Check sheet for the modelled part. Datum: model origin and axes. Units: mm. A direction names the side the tool comes from. Round coordinates to 2 decimals unless told otherwise and drop trailing zeros. Write each loop counter-clockwise with the first axis right and the second up, starting at its lowest first coordinate (ties: lowest second). Pieces come first, ordered by that corner, then holes. Notation, with made-up numbers: (63, 78.5) -> (84, 78.5) arc R22 cw to (84, 84.5) -> close; hole circle Ø4 at (22, 1). An arc over 180 degrees is marked (long way). Write item = value, one per line.
Autodesk Inventor part; units mm, degrees
ref_plane "Work Plane1" through (0, 0, -15) normal (0, 0, 1) x (1, 0, 0)
ref_plane "YZ Plane" through (0, 0, 0) normal (1, 0, 0) x (0, 1, 0)
ref_plane "XZ Plane" through (0, 0, 0) normal (0, 1, 0) x (-1, 0, 0)
sketch "Sketch1" plane through (0, 0, 0) normal (0, 0, 1) x (1, 0, 0)
  line L0 (0, 0) -> (25, 0)
  line L1 (25, 0) -> (25, 40)
  line L2 (25, 40) -> (0, 40)
  line L3 (0, 40) -> (0, 0)
  dimension "d1" = 25
  dimension "d2" = 40
  dimension "d3" = 25
extrude "Extrusion1" add sketch "Sketch1" against normal blind 30
sketch "Sketch2" plane through (25, 0, 0) normal (1, 0, 0) x (0, 0, -1)
  line L0 (0, 0) -> (30, 0)
  circle A0 centre (15, 6.56) radius 2.46
extrude "Extrusion2" cut sketch "Sketch2" against normal blind 30
sketch "Sketch3" plane through (0, 0, 0) normal (-1, 0, 0) x (0, 0, 1)
  line L0 (0, 0) -> (-30, 0)
  line L1 (-25.05, 0) -> (-4.95, 0)
  line L2 (-4.95, 0) -> (-4.95, 33.12)
  line L3 (-4.95, 33.12) -> (-25.05, 33.12)
  line L4 (-25.05, 33.12) -> (-25.05, 0)
  dimension "d11" = 20.1
extrude "Extrusion3" cut sketch "Sketch3" against normal blind 20
sketch "Sketch4" plane through (0, 0, 0) normal (0, -1, 0) x (1, 0, 0)
  line L0 (20, -4.95) -> (20, -25.05)
  line L1 (20, -15) -> (25, -15)
  line L2 (25, 0) -> (25, -30)
  line L3 (20, -8.025) -> (25, -8.025)
  line L4 (25, -8.025) -> (25, -21.975)
  line L5 (25, -21.975) -> (20, -21.975)
  line L6 (20, -21.975) -> (20, -8.025)
  line L7 (20, -8.025) -> (25, -21.975) construction
  line L8 (25, -8.025) -> (20, -21.975) construction
  line L9 (25, -12.54) -> (25, -17.46)
  point P0 (0, 0)
  point P1 (22.5, -15)
  dimension "d14" = 13.95
extrude "Extrusion4" add sketch "Sketch4" along normal blind 15
sketch "Sketch5" plane through (20, 0, 0) normal (-1, 0, 0) x (0, 0, 1)
  circle A0 centre (-15, 6.56) radius 2.46
  circle A1 centre (-15, 6.56) radius 4.7025
  circle A2 centre (-15, 6.56) radius 2.46
  circle A3 centre (-15, 6.56) radius 2.46
  point P0 (0, 0)
  dimension "d17" = 9.405
extrude "Extrusion5" cut sketch "Sketch5" against normal blind 2.1
sketch "Sketch6" plane through (25, 0, 0) normal (1, 0, 0) x (0, 0, -1)
  circle A0 centre (15, 6.56) radius 4.7025
  line L0 (15, 6.56) -> (15, 23.56)
  circle A1 centre (15, 23.56) radius 2.46
  point P0 (0, 0)
  dimension "d20" = 17
  dimension "d21" = 4.92
extrude "Extrusion6" cut sketch "Sketch6" against normal blind 10 contours A1
sketch "Sketch7" plane through (20, 0, 0) normal (-1, 0, 0) x (0, 0, 1)
  circle A0 centre (-15, 23.56) radius 2.46
  circle A1 centre (-15, 23.56) radius 4.7025
  point P0 (0, 0)
  dimension "d24" = 9.405
extrude "Extrusion7" cut sketch "Sketch7" against normal blind 2.1
sketch "Sketch9" plane through (25, 0, 0) normal (1, 0, 0) x (0, 0, -1)
  circle A0 centre (15, 6.56) radius 2.46
  circle A1 centre (15, 6.56) radius 2.46
  circle A2 centre (15, 23.56) radius 2.46
  circle A3 centre (15, 23.56) radius 2.46
  line L0 (30, 40) -> (30, 0)
  line L1 (30, 0) -> (30, 40)
  line L2 (30, 40) -> (0, 40)
  line L3 (0, 40) -> (0, 0)
  line L4 (0, 0) -> (8.025, 0)
  line L5 (21.975, 0) -> (21.975, -15)
  line L6 (21.975, -15) -> (8.025, -15)
  line L7 (8.025, -15) -> (8.025, 0)
  line L8 (0, 0) -> (8.025, 0)
  line L9 (21.975, 0) -> (30, 0)
extrude "Extrusion8" add sketch "Sketch9" along normal blind 5
sketch "Sketch10" plane through (0, 40, 0) normal (0, 1, 0) x (1, 0, 0)
  line L0 (0, 30) -> (30, 30)
  line L1 (30, 0) -> (0, 0)
  line L2 (0, 30) -> (30, 30)
  line L3 (30, 30) -> (30, 0)
  line L4 (30, 0) -> (0, 0)
  line L5 (0, 0) -> (0, 30)
extrude "Extrusion9" add sketch "Sketch10" along normal blind 30
sketch "Sketch12" plane through (30, 0, 0) normal (1, 0, 0) x (0, 0, -1)
  circle A0 centre (15, 6.56) radius 2.46
  line L0 (15, 6.56) -> (15, 15.06)
  circle A1 centre (15, 15.06) radius 2.525
  point P0 (0, 0)
  dimension "d31" = 8.5
  dimension "d33" = 5.05
extrude "Extrusion10" cut sketch "Sketch12" against normal blind 30 contours A1
sketch "Sketch15" plane through (0, 0, -25.05) normal (-1, 0, 0) x (0, 0, 1)
  line L0 (0, 33.12) -> (20.1, 33.12)
  line L1 (20.1, 33.12) -> (20.1, 0)
  line L2 (0, 33.12) -> (20.1, 33.12)
  line L3 (20.1, 33.12) -> (20.1, 31.1)
  line L4 (20.1, 31.1) -> (0, 31.1)
  line L5 (0, 31.1) -> (0, 33.12)
  point P0 (25.05, 0)
  dimension "d57" = 2.02
extrude "Extrusion13" add sketch "Sketch15" against normal blind 20
sketch "Sketch17" plane through (0, 0, 0) normal (0, 0, 1) x (1, 0, 0)
  line L0 (0, 70) -> (30, 70)
  line L1 (30, 70) -> (50.0622, 90.0622)
  line L2 (30, 70) -> (80, 70) construction
  line L3 (11.9522, 97.2454) -> (0, 85.2932)
  line L4 (0, 70) -> (0, 85.2932)
  line L5 (0, 70) -> (0, 0)
  line L6 (0, 70) -> (30, 70)
  line L7 (10.923, 112.2849) -> (0, 120.567)
  line L8 (50.0622, 105.3553) -> (50.0622, 120.567)
  line L9 (50.0622, 105.3553) -> (50.0622, 90.0622)
  arc A0 (11.9522, 97.2454) -> (10.923, 112.2849) centre (4.8811, 104.3165) ccw
  line L10 (4, 138.567) -> (0, 140.567)
  line L11 (4, 122.567) -> (0, 120.567)
  line L12 (4, 122.567) -> (8, 130.567)
  line L13 (4, 138.567) -> (8, 130.567)
  line L14 (0, 140.567) -> (30, 140.567)
  line L15 (30, 140.567) -> (50.0622, 120.567)
  dimension "d61" = 45
  dimension "d62" = 32.0271
  dimension "d72" = 10
extrude "Extrusion14" add sketch "Sketch17" against normal blind 30
sketch "Sketch21" plane through (0, 0, 0) normal (0, 0, 1) x (1, 0, 0)
  line L0 (50.0622, 90.0622) -> (30, 70)
  line L1 (30, 70) -> (50.0622, 90.0622)
  line L2 (50.0622, 90.0622) -> (50.0622, 120.567)
  line L3 (50.0622, 90.0622) -> (50.0622, 120.567)
  line L4 (0, 140.567) -> (30, 140.567)
  line L5 (50.0622, 120.567) -> (30, 140.567)
  line L6 (30, 140.567) -> (0, 140.567)
  line L7 (4, 138.567) -> (0, 140.567)
  line L8 (0, 140.567) -> (4, 138.567)
  line L9 (8, 130.567) -> (4, 138.567)
  line L10 (4, 138.567) -> (8, 130.567)
  line L11 (4, 122.567) -> (8, 130.567)
  line L12 (8, 130.567) -> (4, 122.567)
  line L13 (0, 120.567) -> (4, 122.567)
  line L14 (4, 122.567) -> (0, 120.567)
  line L15 (10.923, 112.2849) -> (0, 120.567)
  line L16 (0, 120.567) -> (10.923, 112.2849)
  line L17 (0, 85.2932) -> (11.9522, 97.2454)
  line L18 (11.9522, 97.2454) -> (0, 85.2932)
  line L19 (0, 85.2932) -> (0, 55.2932)
  line L20 (0, 55.2932) -> (30, 55.2932)
  line L21 (30, 55.2932) -> (30, 70)
  arc A0 (11.9522, 97.2454) -> (10.923, 112.2849) centre (4.8811, 104.3165) ccw
  dimension "d79" = 30
  dimension "d81" = 30
extrude "Extrusion15" add sketch "Sketch21" along normal blind 30
ref_plane "Work Plane1" through (0, 0, -15) normal (0, 0, 1) x (1, 0, 0)
mirror "Mirror1" about plane through (0, 0, -15) normal (0, 0, 1) of "Extrusion15"
properties part number "rec_c_16mm_x_90mm"
(1) Release check for a two-part mould opening along Y. For faces 5 (the flat face through (15, 55.293, -45)), 6 (the flat face through (2.03, 121.58, -14.37)), 7 (the cylindrical face through (25.995, 7.502, -17.272)), 8 (the flat face through (50.062, 106, -14)) record: pulls with the +Y half, pulls with the -Y half, needs draft (parallel to the pull), parting line crosses it, or undercut.
Worked answers:
face_5 = pulls with the -Y half
face_6 = undercut
face_7 = undercut
face_8 = needs draft
(2) Sectioned sample at D-D on z = -38. Enter the section's corners in (x, y).
Worked answers:
outline = (0, 55.29) -> (30, 55.29) -> (30, 70) -> (50.06, 90.06) -> (50.06, 120.57) -> (30, 140.57) -> (0, 140.57) -> (4, 138.57) -> (8, 130.57) -> (4, 122.57) -> (0, 120.57) -> (10.92, 112.28) arc R10 cw to (11.95, 97.25) -> (0, 85.29) -> close
(3) Sectioned sample at A-A on y = 23.56. Enter the section's corners in (x, z), then the cut area to 3 significant figures.
Worked answers:
outline = (0, -30) -> (30, -30) -> (30, -17.46) -> (22.1, -17.46) -> (22.1, -19.7) -> (20, -19.7) -> (20, -25.05) -> (0, -25.05) -> close; (0, -4.95) -> (20, -4.95) -> (20, -10.3) -> (22.1, -10.3) -> (22.1, -12.54) -> (30, -12.54) -> (30, 0) -> (0, 0) -> close
area = 439 mm²
(4) Sectioned sample at B-B on z = -3. Enter the section's corners in (x, y).
Worked answers:
outline = (0, 0) -> (30, 0) -> (30, 70) -> (50.06, 90.06) -> (50.06, 120.57) -> (30, 140.57) -> (0, 140.57) -> (4, 138.57) -> (8, 130.57) -> (4, 122.57) -> (0, 120.57) -> (10.92, 112.28) arc R10 cw to (11.95, 97.25) -> (0, 85.29) -> close
(5) Material ranges on L1, parallel to Y at x = 27.5, z = -15 (3 decimals); L2, parallel to Y at x = 3.5, z = -12; L3, parallel to X at y = 64, z = -1.5, recorded low to high. Write a range as [from, to].
Worked answers:
L1 = [-15, 4.1], [9.02, 12.535], [17.585, 21.1], [26.02, 140.567]
L2 = [31.1, 88.79], [117.91, 122.32], [138.82, 140.57]
L3 = [0, 30]
(6) Go/stop test with flat-tipped pins: P1, Ø4, axis at x = 8.5, z = -2.5, coming from the -Y side; P2, Ø4.5, axis at y = 25.5, z = -17, coming from the -X side; P3, Ø24, axis at x = 15.5, y = 30, coming from the -Z side; P4, Ø10, axis at x = 33, z = -14, coming from the -Y side. Record where each tip stops, or that it passes through.
Worked answers:
P1 = 0
P2 = 20
P3 = -30
P4 = -15
(7) Access from +Z, -Z, +X, -X, +Y, -Y to the whole of each face (thin tool, end or side, straight path). Record for faces 1 (the flat face through (6.06, 91.353, -14.37)), 2 (the flat face through (25, -7, -21.975)), 3 (the flat face through (30, 47, -14)), 4 (the flat face through (20, 8, -20)).
Worked answers:
face_1 = +Z, -Z, -X
face_2 = -Z, +X, -X, -Y
face_3 = +Z, -Z, +X, -Y
face_4 = -X, -Y
(8) Sectioned sample at C-C on x = 26. Enter the section's corners in (y, z) (3 decimals).
Worked answers:
outline = (-15, -21.975) -> (0, -21.975) -> (0, -30) -> (55.293, -30) -> (55.293, -60) -> (140.567, -60) -> (140.567, 30) -> (55.293, 30) -> (55.293, 0) -> (0, 0) -> (0, -8.025) -> (-15, -8.025) -> close; hole circle Ø4.92 at (6.56, -15); hole circle Ø5.05 at (15.06, -15); hole circle Ø4.92 at (23.56, -15)
